Can you work these out from the drawing? Everything is in mm from the part's minimum corner. A direction names the side the tool comes from. Give positions to 0.01 mm unless a question says otherwise; leave off trailing zeros. Loops run counter-clockwise (first coordinate to the right, second up) from the corner with the lowest first, then second, coordinate; pieces in that order, holes last. Notation, with made-up numbers: (-8.5, 83.5) - (3.5, 83.5) arc R21 cw to (3.5, 121.5) - close; hole circle Ø11 at (-33.5, 80). An arc over 180 degrees is marked (long way). Answer in a Markdown table with one row per item.
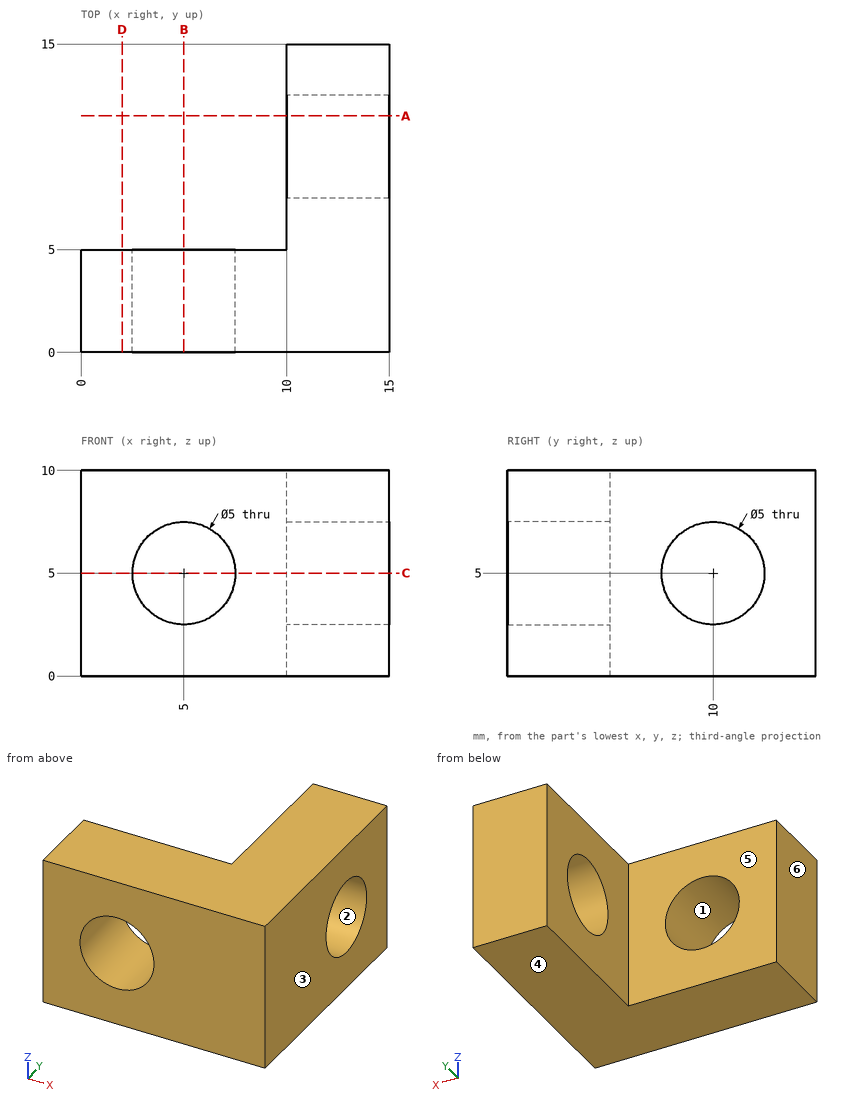
Q1. For pin 1 (1 mm diameter, centred on y = 13.5, z = 8, fed in from -X), with a flat end and sliding along its axis, tell me the tip position at first contact or that it passes through.
Checked values:
| item | result |
|---|---|
| pin 1 | stops at x = 10 |
Q2. Imagine slicing it at A-A, the plane y = 11.5. Write out the boundary of the cut face in (x, z), and give its area (3 significant figures).
Checked values:
| item | result |
|---|---|
| outline | (10, 0) - (15, 0) - (15, 3) - (10, 3) - close; (10, 7) - (15, 7) - (15, 10) - (10, 10) - close |
| area | 30.0 mm² |
Q3. If I drill on line 1 (Y direction, x = 12.05, z = 5); line 2 (X direction, y = 2.65, z = 5); line 3 (X direction, y = 13.5, z = 7.25), over which ranges is the centre line in solid material (lowest first)? Write a range as [from, to].
Checked values:
| item | result |
|---|---|
| line 1 | y = [0, 7.5], [12.5, 15] |
| line 2 | x = [0, 2.5], [7.5, 15] |
| line 3 | x = [10, 15] |
Q4. On a 3-axis mill with a long thin cutter (end or side, diameter ignored), from which of +Z, -Z, +X, -X, +Y, -Y can I reach the whole of each face in a straight line? I mean the marked faces 5 and 6. Say none if no direction works.
Checked values:
| item | result |
|---|---|
| face 5 | +Z, -Z, -X, +Y |
| face 6 | +Z, -Z, -X, +Y, -Y |
Q5. Imagine slicing it at D-D, the plane x = 2. Write out the boundary of the cut face in (y, z), and give its area (3 significant figures).
Checked values:
| item | result |
|---|---|
| outline | (0, 0) - (5, 0) - (5, 10) - (0, 10) - close |
| area | 50.0 mm² |
Q6. If we mould it in two halves opening along Z, with no side actions, what happens to the marked faces 1, 2, 3 and 4? For each: released by +Z, released by -Z, zero draft, split by the parting line, or undercut.
Checked values:
| item | result |
|---|---|
| face 1 | undercut |
| face 2 | undercut |
| face 3 | zero draft |
| face 4 | released by -Z |
Q7. Imagine slicing it at B-B, the plane x = 5. Write out the boundary of the cut face in (y, z).
Checked values:
| item | result |
|---|---|
| outline | (0, 0) - (5, 0) - (5, 2.5) - (0, 2.5) - close; (0, 7.5) - (5, 7.5) - (5, 10) - (0, 10) - close |
Q8. Imagine slicing it at C-C, the plane z = 5. Write out the boundary of the cut face in (x, y).
Checked values:
| item | result |
|---|---|
| outline | (0, 0) - (2.5, 0) - (2.5, 5) - (0, 5) - close; (7.5, 0) - (15, 0) - (15, 7.5) - (10, 7.5) - (10, 5) - (7.5, 5) - close; (10, 12.5) - (15, 12.5) - (15, 15) - (10, 15) - close |
